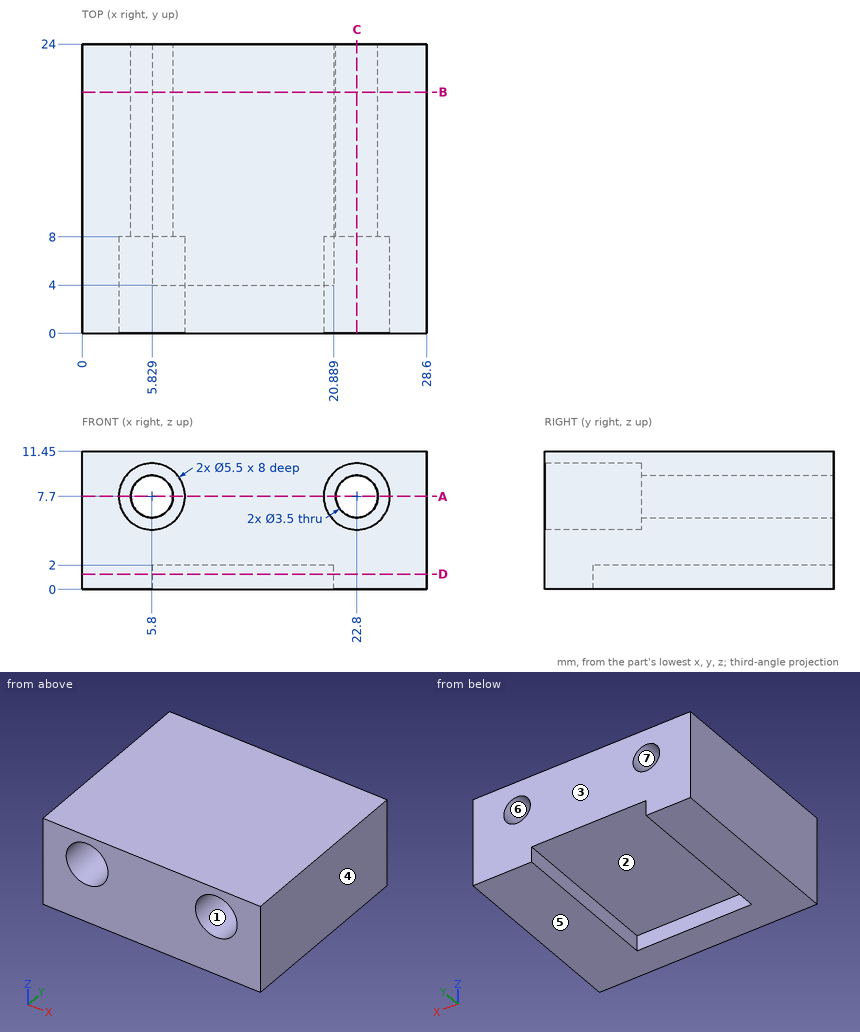
For this review, use the dimensioned drawing (mm, ordinates from the lowest corner) and the shaded views. A direction names the side the tool comes from. Coordinates: 2 decimals unless noted, no trailing zeros. Loops run counter-clockwise (first coordinate to the right, second up) from the corner with the lowest first, then second, coordinate; pieces in that order, holes last. Notation, with made-up numbers: (7, 69) -> (62, 69) arc R28 cw to (62, 106) -> close; hole circle Ø11 at (-14, 34). An arc over 180 degrees is marked (long way). Return JSON: item names as keys, results as strings. Group by question number.
(1) To check wall thickness, follow L1, parallel to X at y = 1.5, z = 7.75; L2, parallel to Z at x = 22.8, y = 2.5; L3, parallel to Y at x = 17.75, z = 1.5. State the ranges of each line that lie inside material, in increasing order.
(2) For pin 1 Ø7.5 at (x, y) = (14.5, 15) entering from -Z; pin 2 Ø5 at (x, z) = (5.8, 7.7) entering from -Y; pin 3 Ø3 at (x, z) = (5.8, 7.7) entering from -Y; pin 4 Ø0.6 at (x, z) = (13, 1.5) entering from +Y, all flat-tipped, find the tip position at first contact; note any pin that passes through.
(3) Tool access review of the marked faces 1, 2 and 3: name each direction out of +Z, -Z, +X, -X, +Y, -Y from which nothing blocks a thin tool from reaching the whole face with its end or side.
(4) Consider section A-A, the plane z = 7.7. Give the boundary of the cut face in (x, y).
(5) Consider section C-C, the plane x = 22.8. Give the boundary of the cut face in (y, z).
(6) Consider section B-B, the plane y = 20. Give the boundary of the cut face in (x, z).
(7) Mouldability with a two-part tool opening along Z and no side actions: class the marked faces 4, 5, 6 and 7 as pulls with the +Z half, pulls with the -Z half, needs draft (parallel to the pull), parting line crosses it, or undercut.
(8) Consider section D-D, the plane z = 1.25. Give the boundary of the cut face in (x, y), plus the area to 3 significant figures.
Results below:
{
 "1": {"L1": "x = 0 to 3.05, 8.55 to 20.05, 25.55 to 28.6", "L2": "z = 0 to 4.95, 10.45 to 11.45", "L3": "y = 0 to 4"},
 "2": {"pin 1": "stops at z = 2", "pin 2": "stops at y = 8", "pin 3": "passes through", "pin 4": "stops at y = 4"},
 "3": {"face 1": "-Y", "face 2": "-Z, +Y", "face 3": "+Z, -Z, +X, -X, +Y"},
 "4": {"outline": "(0, 0) -> (3.05, 0) -> (3.05, 8) -> (4.05, 8) -> (4.05, 24) -> (0, 24) -> close; (7.55, 8) -> (8.55, 8) -> (8.55, 0) -> (20.05, 0) -> (20.05, 8) -> (21.05, 8) -> (21.05, 24) -> (7.55, 24) -> close; (24.55, 8) -> (25.55, 8) -> (25.55, 0) -> (28.6, 0) -> (28.6, 24) -> (24.55, 24) -> close"},
 "5": {"outline": "(0, 0) -> (24, 0) -> (24, 5.95) -> (8, 5.95) -> (8, 4.95) -> (0, 4.95) -> close; (0, 10.45) -> (8, 10.45) -> (8, 9.45) -> (24, 9.45) -> (24, 11.45) -> (0, 11.45) -> close"},
 "6": {"outline": "(0, 0) -> (5.83, 0) -> (5.83, 2) -> (20.89, 2) -> (20.89, 0) -> (28.6, 0) -> (28.6, 11.45) -> (0, 11.45) -> close; hole circle Ø3.5 at (5.8, 7.7); hole circle Ø3.5 at (22.8, 7.7)"},
 "7": {"face 4": "needs draft", "face 5": "pulls with the -Z half", "face 6": "undercut", "face 7": "undercut"},
 "8": {"outline": "(0, 0) -> (28.6, 0) -> (28.6, 24) -> (20.89, 24) -> (20.89, 4) -> (5.83, 4) -> (5.83, 24) -> (0, 24) -> close", "area": "385 mm2"}
}
